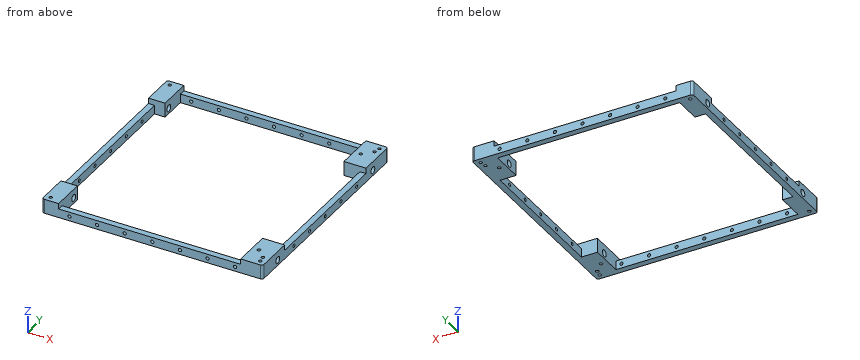
Autodesk Inventor part; units mm, degrees
ref_plane "YZ Plane" through (0, 0, 0) normal (1, 0, 0) x (0, 1, 0)
ref_plane "XZ Plane" through (0, 0, 0) normal (0, 1, 0) x (-1, 0, 0)
ref_plane "XY Plane" through (0, 0, 0) normal (0, 0, 1) x (1, 0, 0)
ref_plane "Work Plane1" through (181.6, 41.8, 16) normal (0, 0, -1) x (-1, 0, 0)
sketch "Sketch1" plane through (181.6, 41.8, 16) normal (0, 0, -1) x (-1, 0, 0)
  circle A0 centre (0.9, -0.9) radius 1.45 construction
  line L0 (4, -1.5) -> (1.5, -4) construction
  line L1 (4, -1.5) -> (4, 4) construction
  line L2 (4, 4) -> (-2, 4) construction
  arc A1 (-2, 4) -> (-4, 2) centre (-2, 2) ccw construction
  line L3 (-4, 2) -> (-4, -4) construction
  line L4 (-4, -4) -> (1.5, -4) construction
  arc A2 (45.8, 2) -> (43.8, 4) centre (43.8, 2) ccw construction
  line L5 (43.8, 4) -> (37.8, 4) construction
  line L6 (37.8, 4) -> (37.8, -1.5) construction
  line L7 (40.3, -4) -> (45.8, -4) construction
  line L8 (45.8, -4) -> (45.8, 2) construction
  circle A3 centre (40.9, -0.9) radius 1.45 construction
  line L9 (37.8, -40.3) -> (40.3, -37.8) construction
  line L10 (37.8, -40.3) -> (37.8, -45.8) construction
  line L11 (37.8, -45.8) -> (43.8, -45.8) construction
  arc A4 (43.8, -45.8) -> (45.8, -43.8) centre (43.8, -43.8) ccw construction
  line L12 (45.8, -43.8) -> (45.8, -37.8) construction
  line L13 (45.8, -37.8) -> (40.3, -37.8) construction
  circle A5 centre (40.9, -40.9) radius 1.45 construction
  circle A6 centre (0.9, -40.9) radius 1.45 construction
  line L14 (1.5, -37.8) -> (4, -40.3) construction
  line L15 (1.5, -37.8) -> (-4, -37.8) construction
  line L16 (-4, -37.8) -> (-4, -43.8) construction
  arc A7 (-4, -43.8) -> (-2, -45.8) centre (-2, -43.8) ccw construction
  line L17 (-2, -45.8) -> (4, -45.8) construction
  line L18 (4, -45.8) -> (4, -40.3) construction
  line L19 (40.3, -4) -> (37.8, -1.5) construction
  line L20 (-52, 154) -> (143.8, 154)
  line L21 (145.8, 152) -> (145.8, -43.8)
  line L22 (143.8, -45.8) -> (-52, -45.8)
  line L23 (-54, -43.8) -> (-54, 152)
  line L24 (140.3, -37.8) -> (140.3, 146)
  line L25 (137.8, 148.5) -> (-46, 148.5)
  line L26 (-48.5, 146) -> (-48.5, -37.8)
  line L27 (-46, -40.3) -> (137.8, -40.3)
  line L28 (137.8, -40.3) -> (140.3, -37.8)
  line L29 (-46, -40.3) -> (-48.5, -37.8)
  line L30 (-46, 148.5) -> (-48.5, 146)
  line L31 (140.3, 146) -> (137.8, 148.5)
  arc A8 (145.8, 152) -> (143.8, 154) centre (143.8, 152) ccw
  arc A9 (143.8, -45.8) -> (145.8, -43.8) centre (143.8, -43.8) ccw
  arc A10 (-54, -43.8) -> (-52, -45.8) centre (-52, -43.8) ccw
  arc A11 (-52, 154) -> (-54, 152) centre (-52, 152) ccw
  circle A12 centre (140.8, -40.8) radius 1.4
  circle A13 centre (-49, -40.8) radius 1.4
  circle A14 centre (45.9, 54.1) radius 94.4 construction
  line L32 (45.9, 148.5) -> (45.9, -40.3)
  line L33 (77.4, 111.7) -> (64.2, 111.7) construction
  line L34 (64.2, 96.7) -> (77.4, 96.7) construction
  line L35 (77.4, 61.7) -> (64.2, 61.7) construction
  line L36 (64.2, 46.7) -> (77.4, 46.7) construction
  circle A15 centre (140.8, 149) radius 1.4
  circle A16 centre (-49, 149) radius 1.4
  point P0 (145.8, -45.8)
  point P1 (145.8, 154)
  point P2 (-54, -45.8)
  point P3 (140.3, -40.3)
  point P4 (140.3, 148.5)
  point P5 (-48.5, 148.5)
  point P6 (-48.5, -40.3)
  point P7 (40.8, 149)
  point P8 (45.8, -40.8)
  point P9 (70.9, 96)
  dimension "d34" = 199.8
  dimension "d35" = 199.8
  dimension "d36" = 5.5
  dimension "d37" = 2.5
  dimension "d38" = 2.5
  dimension "d39" = 2.5
  dimension "d40" = 2.5
  dimension "d41" = 2.5
  dimension "d42" = 2.5
  dimension "d43" = 2.5
  dimension "d44" = 2.5
  dimension "d45" = 2
  dimension "d46" = 5
  dimension "d47" = 5
  dimension "d48" = 5
  dimension "d49" = 5
  dimension "d51" = 5
  dimension "d57" = 2.8
  dimension "d58" = 2.8
  dimension "d255" = 2.8
  dimension "d256" = 5
  dimension "d257" = 5
  dimension "d308" = 2.8
  dimension "d309" = 5
  dimension "d310" = 5
extrude "Extrusion1" add sketch "Sketch1" along normal blind 8
sketch "Sketch56" plane through (181.6, 41.8, 8) normal (0, 0, -1) x (-1, 0, 0)
  line L0 (137.8, 148.5) -> (140.3, 146)
  line L1 (140.3, 146) -> (140.3, -37.8) construction
  line L2 (140.3, -37.8) -> (137.8, -40.3)
  line L3 (137.8, -40.3) -> (-46, -40.3)
  line L4 (-46, -40.3) -> (-48.5, -37.8)
  line L5 (-48.5, -37.8) -> (-48.5, 146)
  line L6 (-48.5, 146) -> (-46, 148.5)
  line L7 (-46, 148.5) -> (137.8, 148.5)
  line L8 (145.8, 152) -> (145.8, -43.8)
  arc A0 (143.8, -45.8) -> (145.8, -43.8) centre (143.8, -43.8) ccw
  line L9 (143.8, -45.8) -> (-52, -45.8)
  arc A1 (-54, -43.8) -> (-52, -45.8) centre (-52, -43.8) ccw
  line L10 (-54, -43.8) -> (-54, 152)
  arc A2 (-52, 154) -> (-54, 152) centre (-52, 152) ccw
  line L11 (-52, 154) -> (143.8, 154)
  arc A3 (145.8, 152) -> (143.8, 154) centre (143.8, 152) ccw
  circle A4 centre (140.8, -40.8) radius 1.4
  circle A5 centre (-49, -40.8) radius 1.4
  circle A6 centre (140.8, 149) radius 1.4
  circle A7 centre (-49, 149) radius 1.4
  line L12 (137.8, 148.5) -> (-46, 148.5)
  line L13 (-46, 148.5) -> (-48.5, 146)
  line L14 (-48.5, 146) -> (-48.5, -37.8)
  line L15 (-48.5, -37.8) -> (-46, -40.3)
  line L16 (-46, -40.3) -> (137.8, -40.3)
  line L17 (137.8, -40.3) -> (140.3, -37.8)
  line L18 (140.3, -37.8) -> (140.3, 146)
  line L19 (140.3, 146) -> (137.8, 148.5)
  line L20 (145.8, -45.8) -> (125.8, -45.8) construction
  line L21 (125.8, -45.8) -> (125.8, -15.8) construction
  line L22 (125.8, -15.8) -> (145.8, -15.8) construction
  line L23 (145.8, -15.8) -> (145.8, -45.8) construction
  line L24 (-54, -45.8) -> (-34, -45.8) construction
  line L25 (-34, -45.8) -> (-34, -10.8) construction
  line L26 (-34, -10.8) -> (-54, -10.8) construction
  line L27 (-54, -10.8) -> (-54, -45.8) construction
  line L28 (145.8, -15.8) -> (130.8, -15.8)
  line L29 (130.8, -15.8) -> (130.8, -45.8)
  line L30 (-54, -10.8) -> (-34, -10.8)
  line L31 (-34, -45.8) -> (-34, -10.8)
  line L32 (145.8, -15.8) -> (145.8, -43.8)
  line L33 (143.8, -45.8) -> (130.8, -45.8)
  line L34 (-54, -10.8) -> (-54, -43.8)
  line L35 (-34, -45.8) -> (-52, -45.8)
  point P0 (181.6, -41.8)
  dimension "d373" = 20
  dimension "d374" = 30
  dimension "d375" = 20
  dimension "d376" = 35
  dimension "d377" = 15
extrude "Extrusion35" add sketch "Sketch56" against normal blind 13 contours L28 L8 A0 L9 L29 L3 L2 L18 | L18 L2 L3 L29 L28 | L30 L31 L3 L4 L5 | L5 L4 L3 L31 L9 A1 L10 L30
sketch "Sketch57" plane through (235.6, -2, 16) normal (1, 0, 0) x (0, 0, -1)
  circle A0 centre (3, 22) radius 3.05
  line L0 (8, 195.8) -> (8, 0)
  line L1 (0, 195.8) -> (8, 195.8)
  line L2 (0, 33) -> (0, 195.8)
  line L3 (0, 33) -> (-5, 33)
  line L4 (-5, 0) -> (-5, 33)
  line L5 (8, 0) -> (-5, 0)
  line L6 (8, -2) -> (-5, -2)
  point P0 (16, 2)
  dimension "d379" = 5
  dimension "d380" = 24
extrude "Extrusion36" cut sketch "Sketch57" against normal through all contours A0
sketch "Sketch59" plane through (181.6, 41.8, 21) normal (0, 0, 1) x (1, 0, 0)
  circle A0 centre (40, -27.1) radius 3.5
  line L0 (54, -43.8) -> (54, -10.8)
  line L1 (-170.0796, -30.6) -> (49.9204, -30.6) construction
  line L2 (-170.0796, -30.6) -> (49.9204, -30.6) construction
  arc A1 (-171.5, -32.6) -> (-168.5, -32.6) centre (-170, -34.6) ccw
  circle A2 centre (-170, -34.6) radius 4
  circle A3 centre (48, -35.1) radius 3.5
  line L3 (-170, -38.6) -> (63.6932, -38.6) construction
  line L4 (-170, -38.6) -> (63.6932, -38.6) construction
  point P0 (-181.6, -41.8)
  dimension "d385" = 8
  dimension "d378" = 7
  dimension "d381" = 14
  dimension "d383" = 220
  dimension "d384" = 0
  dimension "d386" = 4
  dimension "d387" = 7
  dimension "d388" = 8
  dimension "d389" = 8
  dimension "d397" = 0
hole "Hole12" at (229.6, 6.7, 21) at (221.6, 14.7, 21) direction (0, 0, -1) diameter 2.9 end through all
sketch "Sketch60" plane through (37.8, -4, 16) normal (0, 1, 0) x (1, 0, 0)
  line L0 (6, 0) -> (189.8, 0)
  line L1 (6, 0) -> (6, 8)
  line L2 (189.8, 8) -> (6, 8)
  line L3 (189.8, 0) -> (189.8, 8)
  circle A0 centre (172.8, 4) radius 1.45
  circle A1 centre (43.1531, 4) radius 1.45
  line L4 (197.8, 0) -> (197.8, 8)
  circle A2 centre (147.8, 4) radius 1.45
  circle A3 centre (122.8, 4) radius 1.45
  circle A4 centre (97.8, 4) radius 1.45
  circle A5 centre (72.8, 4) radius 1.45
  circle A6 centre (47.8, 4) radius 1.45
  circle A7 centre (22.8, 4) radius 1.45
  point P0 (-37.8, 16)
  dimension "d398" = 2.9
  dimension "d399" = 2.9
  dimension "d400" = 25
  dimension "d401" = 4
  dimension "d404" = 25
hole "Hole13" at (210.6, -4, 12) at (185.6, -4, 12) at (160.6, -4, 12) at (135.6, -4, 12) at (110.6, -4, 12) at (85.6, -4, 12) at (60.6, -4, 12) direction (0, 1, 0) diameter 2.9 end through all
sketch "Sketch61" plane through (235.6, -2, 8) normal (1, 0, 0) x (0, 0, -1)
  line L0 (0, 195.8) -> (0, 0)
  line L1 (0, 33) -> (-8, 33)
  line L2 (-8, 189.8) -> (-8, 33)
  line L3 (-8, 189.8) -> (0, 189.8)
  line L4 (0, 33) -> (0, 189.8)
  circle A0 centre (-4, 172.8) radius 1.45
  line L5 (-8, 197.8) -> (0, 197.8)
  circle A1 centre (-4, 147.8) radius 1.45
  circle A2 centre (-4, 122.8) radius 1.45
  circle A3 centre (-4, 97.8) radius 1.45
  circle A4 centre (-4, 72.8) radius 1.45
  circle A5 centre (-4, 47.8) radius 1.45
  point P0 (8, 2)
  dimension "d416" = 2.9
  dimension "d417" = 25
  dimension "d420" = 25
hole "Hole14" at (235.6, 45.8, 12) at (235.6, 70.8, 12) at (235.6, 95.8, 12) at (235.6, 120.8, 12) at (235.6, 145.8, 12) at (235.6, 170.8, 12) direction (-1, 0, 0) diameter 2.9 end through all
ref_plane "Work Plane15" through (50.8, 95.9, 16) normal (0, 1, 0) x (1, 0, 0)
mirror "Mirror3" about plane through (50.8, 95.9, 16) normal (0, 1, 0) of "Extrusion35", "Extrusion36", "Hole12"
properties part number "30_CUBE_openSIM_base_v3"
Geometry check sheet. Reference: the model listing, model coordinates, mm. Coordinates: 2 decimals unless noted, no trailing zeros. Order: outer loops, then holes, each group sorted by start corner. A loop starts at its lowest first (then second) coordinate and runs counter-clockwise, first axis right, second up. Notation, with made-up numbers: M 62,-17.5 L 116,-17.5 A38 ccw 116,21.5 Z; hole C 67.25,42 d6. An arc over 180 degrees is marked long. Use CSV: the item, a comma, the result in double quotes.
Item 1: Cross-section at B-B on x = 190. Record the cut outline in (y, z).
Returned:
outline,"M -4,8 L 1.5,8 L 1.5,16 L -4,16 Z; M 190.3,8 L 195.8,8 L 195.8,16 L 190.3,16 Z"
Item 2: Cross-section at C-C on y = 113.5. Record the cut outline in (x, z).
Returned:
outline,"M 35.8,8 L 41.3,8 L 41.3,16 L 35.8,16 Z; M 230.1,8 L 235.6,8 L 235.6,16 L 230.1,16 Z"
Item 3: Thickness scan on line 1 along Y through (x, z) = (223.5, 18.75); line 2 along Y through (x, z) = (228.5, 13); line 3 along Y through (x, z) = (155, 14.25). Record the ranges inside material, lowest first.
Returned:
line 1,"y = -4 to 31, 160.8 to 195.8"
line 2,"y = -4 to 5.76, 7.64 to 16.95, 23.05 to 31, 160.8 to 168.75, 174.85 to 184.16, 186.04 to 195.8"
line 3,"y = -4 to 1.5, 190.3 to 195.8"
Item 4: Cross-section at A-A on y = 20. Record the cut outline in (x, z), then the cut area to 4 significant figures.
Returned:
outline,"M 35.8,8 L 50.8,8 L 50.8,9.95 L 35.8,9.95 Z; M 35.8,16.05 L 50.8,16.05 L 50.8,21 L 35.8,21 Z; M 215.6,8 L 235.6,8 L 235.6,9.95 L 215.6,9.95 Z; M 215.6,16.05 L 235.6,16.05 L 235.6,21 L 215.6,21 Z"
area,"241.5 mm2"
Item 5: Gauge pin test, flat end, axial feed: pin 1 Ø6 at (x, y) = (39, 80) entering from +Z. Record the tip position at first contact, or that the pin passes through.
Returned:
pin 1,"stops at z = 16"
